from build123d import *

# Parameters (mm, degrees)
F1_DEPTH = 25


# Not quite as in the source:
# - ends of sketch curves that miss each other by under 0.0002 mm in the source are joined


with BuildPart() as f1:
    # F0 (on Front) → F1 (new body)
    with BuildSketch(Plane.XZ):
        with BuildLine():
            ThreePointArc((-170.642238, -2.693902), (-124.029000476, 50.3717259287), (-152.294215, -14.357189))
            Line((-152.294215, -14.357189), (-6.118396, -160.533008))
            ThreePointArc((-6.118396, -160.533008), (10.1027713817, -171.3716456256), (29.236943, -175.177669))
            Line((29.236943, -175.177669), (275.511113, -175.177669))
            ThreePointArc((275.511113, -175.177669), (303.22749884, -156.6581722976), (296.7243169356, -123.9644660644))
            Line((296.7243169356, -123.9644660644), (26.871503, 145.888348))
            ThreePointArc((26.871503, 145.888348), (-5.5708317635, 167.5656232511), (-43.839175, 175.17767))
            Line((-43.839175, 175.17767), (-275.511114, 175.17767))
            ThreePointArc((-275.511114, 175.17767), (-300.7842187682, 161.3415239766), (-302.7451656672, 132.5956816918))
            Line((-302.7451656672, 132.5956816918), (-262.960739, 46.481221))
            ThreePointArc((-262.960739, 46.481221), (-251.37881686, 30.6136107366), (-234.5779690393, 20.4325748914))
            Line((-234.5779690393, 20.4325748914), (-170.642238, -2.693902))
        make_face()
    extrude(amount=F1_DEPTH)


solid = f1.part
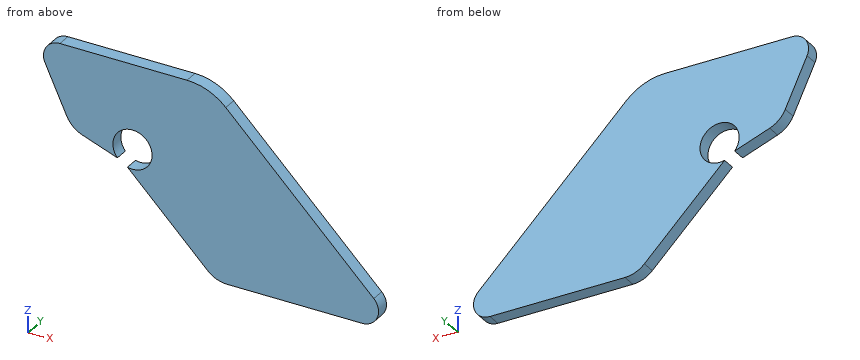
Work out the finished part from the listing and answer in its coordinate system (mm). Give positions to 0.01 mm unless a question says otherwise; leave off trailing zeros. Order: outer loops, then holes, each group sorted by start corner. A loop starts at its lowest first (then second) coordinate and runs counter-clockwise, first axis right, second up. Notation, with made-up numbers: (44.5, -17) -> (50.5, -17) arc R28 cw to (50.5, 22) -> close; hole circle Ø2 at (-32.75, -1.5). An arc over 180 degrees is marked (long way). Answer as a JSON object with one key per item and string values. Group by question number.
1. Section C-C on z = 96 is taken. Determine the outline of the cut face in (x, y).
2. Consider line 1 along X through (y, z) = (-22, 42.5); line 2 along Z through (x, y) = (175.5, -14); line 3 along X through (y, z) = (-16.75, 37). Determine where each line is inside the solid, lowest interval first. Write a range as [from, to].
3. Section A-A on y = -3.75 is taken. Determine the outline of the cut face in (x, z).
4. Section B-B on x = -36.5 is taken. Determine the outline of the cut face in (y, z), plus the area to 3 significant figures.
5. Flat-ended cylindrical pins translate along their axes: pin 1 Ø1.5 at (y, z) = (-17.5, 62) entering from +X; pin 2 Ø1.5 at (x, z) = (-53.5, -7.5) entering from +Y; pin 3 Ø4 at (y, z) = (-10.5, 115) entering from -X; pin 4 Ø3 at (x, y) = (-53.5, -11) entering from -Z. Find the tip coordinate at first contact, or state that the pin passes through.
Result sheet:
{
 "1": {"outline": "(-285.84, -25) -> (76.76, -25) -> (76.76, 0) -> (-285.84, 0) -> close"},
 "2": {"line 1": "x = [-260.9, -171.14], [-115.26, 130.26]", "line 2": "z = [-175.18, -2.74]", "line 3": "x = [-257.23, -174.75], [-111.65, 135.76]"},
 "3": {"outline": "(-302.75, 132.6) -> (-262.96, 46.48) arc R50 ccw to (-234.58, 20.43) -> (-170.64, -2.69) arc R35.74 cw (long way) to (-152.29, -14.36) -> (-6.12, -160.53) arc R50 ccw to (29.24, -175.18) -> (275.51, -175.18) arc R30 ccw to (296.72, -123.96) -> (26.87, 145.89) arc R100 ccw to (-43.84, 175.18) -> (-275.51, 175.18) arc R30 ccw to start"},
 "4": {"outline": "(-25, -130.15) -> (0, -130.15) -> (0, 174.91) -> (-25, 174.91) -> close", "area": "7,630 mm^2"},
 "5": {"pin 1": "stops at x = 111.51", "pin 2": "stops at y = 0", "pin 3": "stops at x = -295.54", "pin 4": "stops at z = -114.65"}
}
